Input: part model. Units: mm. Frame: model coordinates. Face numbers are marked on the shaded views. A direction names the side the tool comes from. Coordinates: 2 decimals unless noted, no trailing zeros. Loops run counter-clockwise (first coordinate to the right, second up) from the corner with the lowest first, then second, coordinate; pieces in that order, holes last.
Autodesk Fusion 360 part; units mm, degrees
sketch "Sketch1" plane through (0, 0, 0) normal (0, 1, 0) x (1, 0, 0)
  line L0 (0, 0) -> (105.6, 0)
  line L1 (105.6, 0) -> (105.6, 16.7)
  line L2 (105.6, 16.7) -> (0, 16.7)
  line L3 (0, 16.7) -> (0, 0)
  dimension "d1" = 105.6
  dimension "d2" = 16.7
extrude "Extrude1" add sketch "Sketch1" along normal blind 2
sketch "Sketch2" plane through (0, 2, 0) normal (0, 1, 0) x (-1, 0, 0)
  line L0 (0, -16.7) -> (0, 0)
  line L1 (0, 0) -> (-105.6, 0)
  line L2 (-105.6, 0) -> (-105.6, -16.7)
  line L3 (-105.6, -16.7) -> (0, -16.7)
  line L4 (0, 0) -> (-105.6, 0)
  line L5 (-105.6, 0) -> (-105.6, -16.7)
  line L6 (-105.6, -16.7) -> (0, -16.7)
  line L7 (0, -16.7) -> (0, 0)
  line L8 (-2, -2) -> (-103.6, -2)
  line L9 (-103.6, -2) -> (-103.6, -14.7)
  line L10 (-103.6, -14.7) -> (-2, -14.7)
  line L11 (-2, -14.7) -> (-2, -2)
  dimension "d5" = 2
extrude "Extrude2" add sketch "Sketch2" along normal blind 19.05
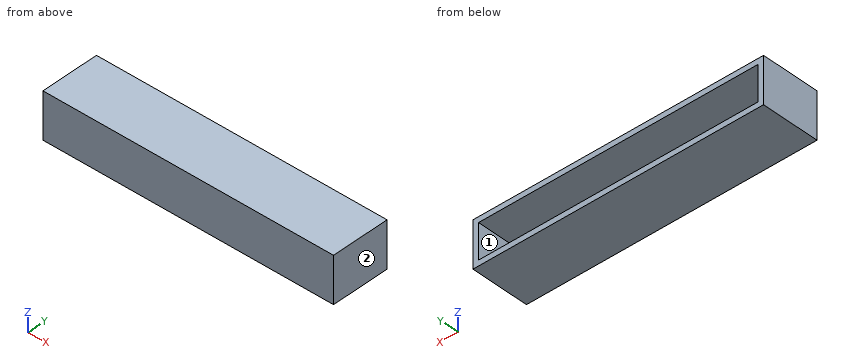
Item 1: Reachability of the marked faces 1 and 2 from +Z, -Z, +X, -X, +Y, -Y: full face, straight path, thin tool, end or side. Return the list, or none.
Result:
face 1: +Y
face 2: +Z, -Z, +X, +Y, -Y
Item 2: Line query: L1, parallel to X at y = 2.75, z = -10.75; L2, parallel to Z at x = 51.5, y = 10; L3, parallel to Y at x = 14, z = -3. Output: solid intervals per line, ascending.
Result:
L1: x = 0 to 2, 103.6 to 105.6
L2: z = -16.7 to -14.7, -2 to 0
L3: y = 0 to 2
Item 3: Section query C-C (x = 92). Output: boundary loops of the cut face in (y, z), then the cut area to 3 significant figures.
Result:
outline: (0, -16.7) - (21.05, -16.7) - (21.05, -14.7) - (2, -14.7) - (2, -2) - (21.05, -2) - (21.05, 0) - (0, 0) - close
area: 110 mm2
Item 4: Contact query for a flat-ended pin moving along its axis: P1, Ø3, axis at x = 88, z = -12.5, coming from the +Y side. Output: stop coordinate, or through.
Result:
P1: stops at y = 2
Item 5: Section query A-A (y = 18.25). Output: boundary loops of the cut face in (x, z).
Result:
outline: (0, -16.7) - (105.6, -16.7) - (105.6, 0) - (0, 0) - close; hole (2, -14.7) - (103.6, -14.7) - (103.6, -2) - (2, -2) - close
Item 6: Section query B-B (z = -11). Output: boundary loops of the cut face in (x, y).
Result:
outline: (0, 0) - (105.6, 0) - (105.6, 21.05) - (103.6, 21.05) - (103.6, 2) - (2, 2) - (2, 21.05) - (0, 21.05) - close
